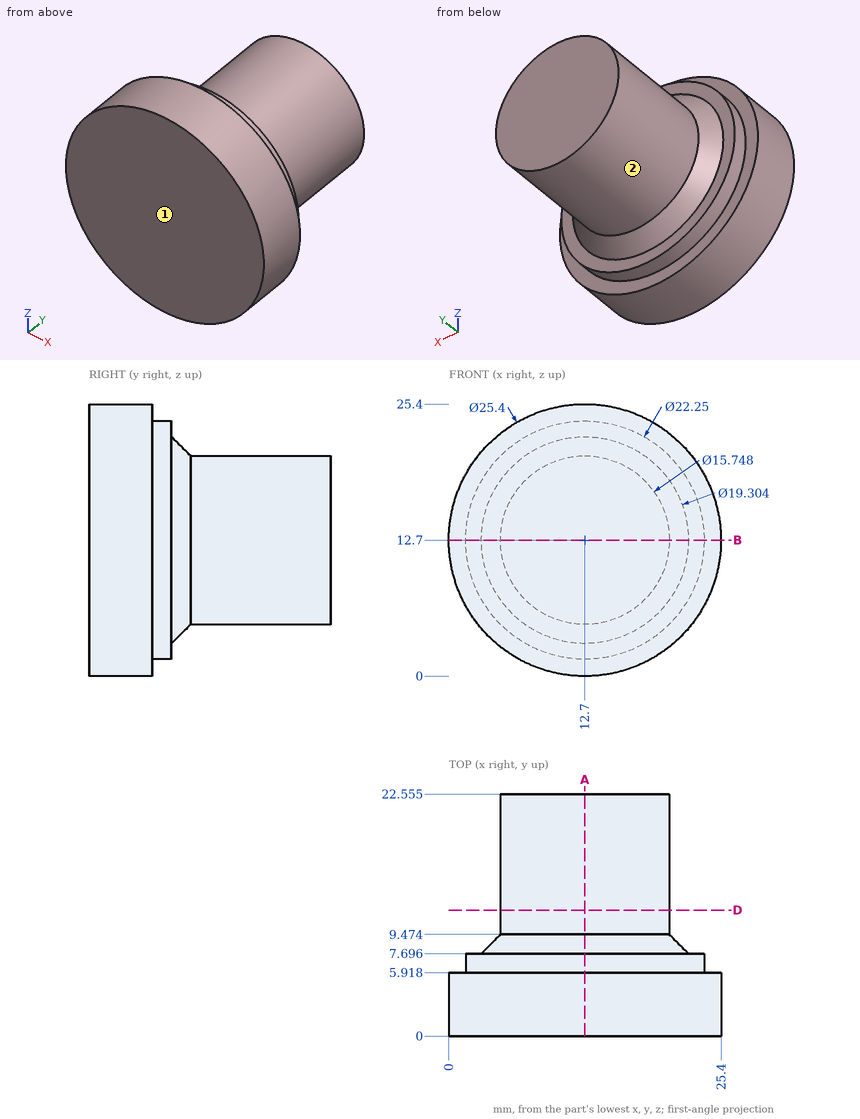
Geometry: see drawing. Coordinates: mm, zero at the bounding-box minimum. A direction names the side the tool comes from. Round coordinates to 2 decimals unless told otherwise and drop trailing zeros. Loops run counter-clockwise (first coordinate to the right, second up) from the corner with the lowest first, then second, coordinate; pieces in that order, holes last.
(1) Access query for the marked faces 1 and 2. Directions: +Z, -Z, +X, -X, +Y, -Y. A direction counts if a zero-diameter tool reaches every point of the face in a straight line with its end or side. Return the directions, or none.
From the geometry:
face 1: +Z, -Z, +X, -X, -Y
face 2: +Y
(2) Section query B-B (z = 12.7). Output: boundary loops of the cut face in (x, y) (1 decimal), and give its area (3 significant figures).
From the geometry:
outline: (0, 0) - (25.4, 0) - (25.4, 5.9) - (23.8, 5.9) - (23.8, 7.7) - (22.4, 7.7) - (20.6, 9.5) - (20.6, 22.6) - (4.8, 22.6) - (4.8, 9.5) - (3, 7.7) - (1.6, 7.7) - (1.6, 5.9) - (0, 5.9) - close
area: 427 mm2
(3) Material intervals for probe 1 along X at (y, z) = (11.5, 13); probe 2 along Y at (x, z) = (19.5, 22); probe 3 along Y at (x, z) = (2.5, 14), sorted ascending.
From the geometry:
probe 1: x = 4.83 to 20.57
probe 2: y = 0 to 5.92
probe 3: y = 0 to 7.7
(4) Section query A-A (x = 12.7). Output: boundary loops of the cut face in (y, z) (1 decimal).
From the geometry:
outline: (0, 0) - (5.9, 0) - (5.9, 1.6) - (7.7, 1.6) - (7.7, 3) - (9.5, 4.8) - (22.6, 4.8) - (22.6, 20.6) - (9.5, 20.6) - (7.7, 22.4) - (7.7, 23.8) - (5.9, 23.8) - (5.9, 25.4) - (0, 25.4) - close
(5) Section query D-D (y = 11.75). Output: boundary loops of the cut face in (x, z).
From the geometry:
outline: circle Ø15.75 at (12.7, 12.7)
(6) Contact query for flat-ended pins moving along their axis: pin 1 Ø5 at (x, z) = (6, 22.5) entering from -Y; pin 2 Ø1.5 at (y, z) = (7, 19.5) entering from +X; pin 3 Ø1.5 at (x, z) = (5, 8) entering from +Y; pin 4 Ø2 at (x, y) = (10.5, 12) entering from +Z. Output: stop coordinate, or through.
From the geometry:
pin 1: stops at y = 0
pin 2: stops at x = 22.04
pin 3: stops at y = 9.08
pin 4: stops at z = 20.48
